```python
from build123d import *

# Parameters (mm, degrees)
BOX_W                         = 1
BOX_H                         = 11
BOX_DEPTH                     = 30
CYLINDER_R                    = 1
CYLINDER_DEPTH                = 20
CYLINDER_PITCH_ANGLE          = 90
CYLINDER003_R                 = 1
CYLINDER003_DEPTH             = 20
CYLINDER003_PITCH_ANGLE       = 90
CYLINDER004001_R              = 2.5
CYLINDER004001_DEPTH          = 7
CYLINDER004001_PITCH_ANGLE    = 90
CYLINDER004_R                 = 3
CYLINDER004_DEPTH             = 7
CYLINDER004_PITCH_ANGLE       = 90
CYLINDER004002_R              = 2.5
CYLINDER004002_DEPTH          = 7
CYLINDER004002_PITCH_ANGLE    = 90
CYLINDER004002001_R           = 3
CYLINDER004002001_DEPTH       = 7
CYLINDER004002001_PITCH_ANGLE = 90
CYLINDER001_R                 = 2.5
CYLINDER001_DEPTH             = 30
CYLINDER002_R                 = 10
CYLINDER002_DEPTH             = 30


with BuildPart() as obj1:
    # Box → Box (new body)
    with BuildSketch(Plane(origin=(-0.5, 0, 0), x_dir=(1, 0, 0), z_dir=(0, 0, 1))):
        with Locations((0.5, 5.5)):
            Rectangle(BOX_W, BOX_H)
    extrude(amount=BOX_DEPTH)


with BuildPart() as trou_vis_haut:
    # Cylinder → Cylinder (new body)
    with BuildSketch(Plane.XY):
        Circle(CYLINDER_R)
    extrude(amount=CYLINDER_DEPTH)


with BuildPart() as trou_vis_haut_1:
    # Cylinder pitch: moved
    add(trou_vis_haut.part.rotate(Axis((0, 0, 0), (0, 1, 0)), CYLINDER_PITCH_ANGLE))


with BuildPart() as trou_vis_haut_2:
    # Cylinder placement: moved
    add(trou_vis_haut_1.part.moved(Location((-10, 5, 23))))


with BuildPart() as trou_vis_bas:
    # Cylinder003 → Cylinder003 (new body)
    with BuildSketch(Plane.XY):
        Circle(CYLINDER003_R)
    extrude(amount=CYLINDER003_DEPTH)


with BuildPart() as trou_vis_bas_1:
    # Cylinder003 pitch: moved
    add(trou_vis_bas.part.rotate(Axis((0, 0, 0), (0, 1, 0)), CYLINDER003_PITCH_ANGLE))


with BuildPart() as trou_vis_bas_2:
    # Cylinder003 placement: moved
    add(trou_vis_bas_1.part.moved(Location((-10, 5, 7))))


with BuildPart() as obj2:
    # Cylinder004001 → Cylinder004001 (new body)
    with BuildSketch(Plane.XY):
        Circle(CYLINDER004001_R)
    extrude(amount=CYLINDER004001_DEPTH)


with BuildPart() as obj2_1:
    # Cylinder004001 pitch: moved
    add(obj2.part.rotate(Axis((0, 0, 0), (0, 1, 0)), CYLINDER004001_PITCH_ANGLE))


with BuildPart() as obj2_2:
    # Cylinder004001 placement: moved
    add(obj2_1.part.moved(Location((-10, 5, 7))))


with BuildPart() as obj3:
    # Cylinder004 → Cylinder004 (new body)
    with BuildSketch(Plane.XY):
        Circle(CYLINDER004_R)
    extrude(amount=CYLINDER004_DEPTH)


with BuildPart() as obj3_1:
    # Cylinder004 pitch: moved
    add(obj3.part.rotate(Axis((0, 0, 0), (0, 1, 0)), CYLINDER004_PITCH_ANGLE))


with BuildPart() as obj3_2:
    # Cylinder004 placement: moved
    add(obj3_1.part.moved(Location((2.999997, 5, 7.000003))))


with BuildPart() as obj4:
    # Cylinder004002 → Cylinder004002 (new body)
    with BuildSketch(Plane.XY):
        Circle(CYLINDER004002_R)
    extrude(amount=CYLINDER004002_DEPTH)


with BuildPart() as obj4_1:
    # Cylinder004002 pitch: moved
    add(obj4.part.rotate(Axis((0, 0, 0), (0, 1, 0)), CYLINDER004002_PITCH_ANGLE))


with BuildPart() as obj4_2:
    # Cylinder004002 placement: moved
    add(obj4_1.part.moved(Location((3, 5, 23))))


with BuildPart() as obj5:
    # Cylinder004002001 → Cylinder004002001 (new body)
    with BuildSketch(Plane.XY):
        Circle(CYLINDER004002001_R)
    extrude(amount=CYLINDER004002001_DEPTH)


with BuildPart() as obj5_1:
    # Cylinder004002001 pitch: moved
    add(obj5.part.rotate(Axis((0, 0, 0), (0, 1, 0)), CYLINDER004002001_PITCH_ANGLE))


with BuildPart() as obj5_2:
    # Cylinder004002001 placement: moved
    add(obj5_1.part.moved(Location((-10, 5, 23))))


with BuildPart() as cylinder001:
    # Cylinder001 → Cylinder001 (new body)
    with BuildSketch(Plane.XY):
        Circle(CYLINDER001_R)
    extrude(amount=CYLINDER001_DEPTH)


with BuildPart() as cut007:
    # Cylinder002 → Cylinder002 (new body)
    with BuildSketch(Plane.XY):
        Circle(CYLINDER002_R)
    extrude(amount=CYLINDER002_DEPTH)

    # Cut: cut Cylinder001
    add(cylinder001.part, mode=Mode.SUBTRACT)

    # Cut001: cut obj5
    add(obj5_2.part, mode=Mode.SUBTRACT)

    # Cut002: cut obj4
    add(obj4_2.part, mode=Mode.SUBTRACT)

    # Cut003: cut obj3
    add(obj3_2.part, mode=Mode.SUBTRACT)

    # Cut004: cut obj2
    add(obj2_2.part, mode=Mode.SUBTRACT)

    # Cut005: cut trou vis bas
    add(trou_vis_bas_2.part, mode=Mode.SUBTRACT)

    # Cut006: cut  trou vis haut
    add(trou_vis_haut_2.part, mode=Mode.SUBTRACT)

    # Cut007: cut obj1
    add(obj1.part, mode=Mode.SUBTRACT)


solid = cut007.part
```
CAD build for the part. Positions are in the model's coordinates, mm. A direction names the side the tool comes from. Coordinates: 2 decimals unless noted, no trailing zeros. Order: outer loops, then holes, each group sorted by start corner. A loop starts at its lowest first (then second) coordinate and runs counter-clockwise, first axis right, second up. Notation, with made-up numbers: (20.25, -10) - (45.25, -10) arc R27 cw to (45.25, 10) - close; hole circle Ø11 at (78.5, -30.5). An arc over 180 degrees is marked (long way). Use a Markdown table: item, result. Add a question column.
(1) Saw through at D-D (x = 8). Give the cut face in (y, z), then the cut area to 3 significant figures.
(2) Drill centre lines: line 1 along Z through (x, y) = (1.85, 5); line 2 along Z through (x, y) = (-7.5, 5); line 3 along Y through (x, z) = (1.4, 7). Where is each one in solid material? Low to high. Write a range as [from, to].
(3) Saw through at B-B (y = -1.25). Give the cut face in (x, z).
(4) Pull direction Z, two halves, no side cores. Call faces 5 (the face through (2, -2, 0)), 6 (the face through (-0.1, -2.5, 14.8)), 7 (the face through (2, -2, 30)), 8 (the face through (1.732, 5.676, 7.737)): +Z half, -Z half, draft (parallel to the pull), parting line (faces both ways), or undercut.
(5) Which spindle directions (+Z, -Z, +X, -X, +Y, -Y) get a long thin tool onto all of the face, cutting with end or side? Do faces 1 (the face through (-5.65, 2.56, 7.54)), 2 (the face through (-2, 6, 7)), 3 (the face through (3, 4, 22)), 4 (the face through (-0.5, 6, 15)). Say none if no direction does.
(6) Saw through at A-A (x = 2). Give the cut face in (y, z), then the cut area to 3 significant figures.
(7) Flat gauge pins, fed straight in: pin 1 (3 mm diameter, centred on y = 5, z = 7, fed in from -X); pin 2 (6 mm diameter, centred on y = 5.5, z = 18.5, fed in from +X); pin 3 (5 mm diameter, centred on y = 5, z = 7, fed in from +X); pin 4 (5 mm diameter, centred on x = -0.5, y = 7, fed in from -Z). Where does each tip first touch, or does it go through?
(8) Saw through at C-C (z = 23.5). Give the cut face in (x, y).
Solved:
| question | item | result |
|---|---|---|
| 1 | outline | (-6, 0) - (6, 0) - (6, 4.17) arc R3 cw (long way) to (6, 9.83) - (6, 20.71) arc R2.5 cw (long way) to (6, 25.29) - (6, 30) - (-6, 30) - close |
| 1 | area | 325 mm² |
| 2 | line 1 | z = [0, 6], [8, 22], [24, 30] |
| 2 | line 2 | z = [0, 4.5], [9.5, 20], [26, 30] |
| 2 | line 3 | y = [-9.9, -2.07], [2.07, 4], [6, 9.9] |
| 3 | outline | (-9.92, 0) - (-2.17, 0) - (-2.17, 30) - (-9.92, 30) - close; (2.17, 0) - (9.92, 0) - (9.92, 30) - (2.17, 30) - close |
| 4 | face 5 | -Z half |
| 4 | face 6 | draft |
| 4 | face 7 | +Z half |
| 4 | face 8 | undercut |
| 5 | face 1 | -X |
| 5 | face 2 | +X, -X |
| 5 | face 3 | +X |
| 5 | face 4 | +Z, -Z, +Y |
| 6 | outline | (-9.8, 0) - (-1.5, 0) - (-1.5, 30) - (-9.8, 30) - close; (1.5, 0) - (9.8, 0) - (9.8, 30) - (1.5, 30) - close; hole circle Ø2 at (5, 7); hole circle Ø2 at (5, 23) |
| 6 | area | 492 mm² |
| 7 | pin 1 | stops at x = -3 |
| 7 | pin 2 | stops at x = 9.68 |
| 7 | pin 3 | stops at x = 3 |
| 7 | pin 4 | stops at z = 0 |
| 8 | outline | (-9.79, 2.04) arc R10 ccw (long way) to (9.67, 2.55) - (3, 2.55) - (3, 4.13) - (0.5, 4.13) - (0.5, 2.45) arc R2.5 cw (long way) to (-0.5, 2.45) - (-0.5, 4.13) - (-3, 4.13) - (-3, 2.04) - close; (-6.06, 7.96) - (-3, 7.96) - (-3, 5.87) - (-0.5, 5.87) - (-0.5, 9.99) arc R10 ccw to start; (0.5, 5.87) - (3, 5.87) - (3, 7.45) - (6.67, 7.45) arc R10 ccw to (0.5, 9.99) - close |
